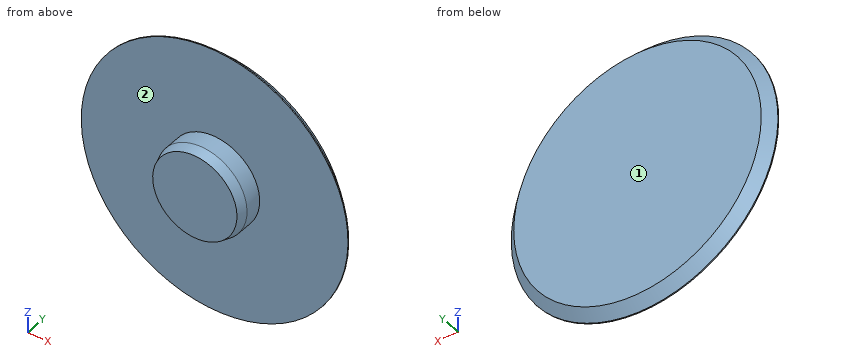
from build123d import *

# Parameters (mm, degrees)
F2_SIZE = 0.9


with BuildPart() as f1:
    # F0 (on Right) → F1 (revolve)
    with BuildSketch(Plane.YZ):
        Polygon((0, 0), (3.5, 0), (3.5, 12.5), (2.5, 12.5), (2.5, 4.225), (0.9, 4.225), (0, 3.95), align=None)
    revolve(axis=Axis((0, 1.75, 0), (0, -1, 0)))

    # F2
    f2_edges = [f1.edges().sort_by_distance(p)[0] for p in [
        (0, 3.5, -12.5),
    ]]
    chamfer(f2_edges, length=F2_SIZE)


solid = f1.part
Can you work these out from the model? Positions are in its coordinate system, mm. Face numbers are marked on the shaded views. A direction names the side the tool comes from. Coordinates: 2 decimals unless noted, no trailing zeros. Write each loop counter-clockwise with the first axis right and the second up, starting at its lowest first coordinate (ties: lowest second). Pieces come first, ordered by that corner, then holes. Notation, with made-up numbers: (-11, -34.75) - (30, -34.75) arc R28 ccw to (30, -0.75) - close; hole circle Ø10 at (19.5, 83). An arc over 180 degrees is marked (long way). Return JSON: item names as keys, results as strings. Group by question number.
Item 1: Which directions (+Z, -Z, +X, -X, +Y, -Y) give clear straight access to the entire face, cutting with the end or side of a thin tool? Please do the marked faces 1 and 2.
Item 2: If we section it at A-A (x = 0): Write out the boundary of the cut face in (y, z) (3 decimals), then the cut area to 3 significant figures.
Item 3: Please list where these lines run through material, in increasing order: probe 1 along Y at (x, z) = (-8.25, 1.75); probe 2 along Z at (x, y) = (-0.25, 1.35); probe 3 along Z at (x, y) = (-2, 2.4).
Item 4: If we section it at C-C (y = 1.95): Write out the boundary of the cut face in (x, z) (3 decimals), then the cut area to 3 significant figures.
Item 5: I'm going to push flat-ended pins straight in: pin 1 Ø1.5 at (x, y) = (8, 2) entering from +Z; pin 2 Ø6 at (x, z) = (-7, -6) entering from -Y. Where does each tip first touch, or does it pass through?
Item 6: If we section it at B-B (z = 0): Write out the boundary of the cut face in (x, y) (3 decimals).
Return value:
{
 "1": {"face 1": "+Z, -Z, +X, -X, +Y", "face 2": "-Y"},
 "2": {"outline": "(0, -3.95) - (0.9, -4.225) - (2.5, -4.225) - (2.5, -12.5) - (2.6, -12.5) - (3.5, -11.6) - (3.5, 11.6) - (2.6, 12.5) - (2.5, 12.5) - (2.5, 4.225) - (0.9, 4.225) - (0, 3.95) - close", "area": "45.1 mm^2"},
 "3": {"probe 1": "y = 2.5 to 3.5", "probe 2": "z = -4.22 to 4.22", "probe 3": "z = -3.72 to 3.72"},
 "4": {"outline": "circle Ø8.45 at (0, 0)", "area": "56.1 mm^2"},
 "5": {"pin 1": "stops at z = 10.04", "pin 2": "stops at y = 2.5"},
 "6": {"outline": "(-12.5, 2.5) - (-4.225, 2.5) - (-4.225, 0.9) - (-3.95, 0) - (3.95, 0) - (4.225, 0.9) - (4.225, 2.5) - (12.5, 2.5) - (12.5, 2.6) - (11.6, 3.5) - (-11.6, 3.5) - (-12.5, 2.6) - close"}
}
